Check sheet for the modelled part. Datum: model origin and axes. Units: mm. A direction names the side the tool comes from. Round coordinates to 2 decimals unless told otherwise and drop trailing zeros. Loops run counter-clockwise (first coordinate to the right, second up) from the corner with the lowest first, then second, coordinate; pieces in that order, holes last. Notation, with made-up numbers: (-35, 10) -> (-29, 10) arc R17 ccw to (-29, 26) -> close; hole circle Ø5 at (35, 13). An arc over 180 degrees is marked (long way). Use one line per item in the form item = value. Start each with the question number.
(1) Sectioned sample at A-A (y = -32.5). Record the cut outline in (x, z), and give its area (3 significant figures).
(2) Material ranges on probe 1 along X at (y, z) = (33.5, 11.75); probe 2 along Z at (x, y) = (-32.65, 36); probe 3 along Y at (x, z) = (-33.05, 14.85), recorded low to high. Write a range as [from, to].
(3) Sectioned sample at C-C (y = 39.5). Record the cut outline in (x, z), and give its area (3 significant figures).
(4) Draft check along Y on faces 1 (the flat face through (33.5, -1, 12)), 2 (the flat face through (-31.5, -1, 13)), 3 (the flat face through (0, -65, 12)). Enter one of: released by +Y, released by -Y, zero draft, split by the parting line, or undercut.
(5) Go/stop test with a flat-tipped pin: pin 1 (0.6 mm diameter, centred on y = -64.5, z = 9.5, fed in from +X). Record where the tip stops, or that it passes through.
(6) Sectioned sample at B-B (x = -2). Record the cut outline in (y, z).
(7) Sectioned sample at D-D (x = 27). Record the cut outline in (y, z), and give its area (3 significant figures).
(8) Set-up check for faces 4 (the cylindrical face through (-32.5, -50.6, 13.8)), 5 (the flat face through (0, 63, 13)), 6 (the flat face through (31, 0, 0)): record each of +Z, -Z, +X, -X, +Y, -Y from which the full face is reachable in a straight line by a thin tool's end or side.
from build123d import *

# Parameters (mm, degrees)
SCHIZZO1_W                    = 67
SCHIZZO1_H                    = 130
ESTRUSIONE_ESTRUSIONE1_DEPTH  = 23
SCHIZZO2_W                    = 63
SCHIZZO2_H                    = 126
TAGLIO_ESTRUSIONE1_DEPTH      = 21
TAGLIO_ESTRUSIONE2_DEPTH      = 77.08054942
TAGLIO_ESTRUSIONE2_DEPTH_BACK = 77.08054942
SCHIZZO3_W                    = 59
SCHIZZO3_H                    = 122
TAGLIO_ESTRUSIONE4_REACH      = 98.141
SCHIZZO4_R                    = 1.5
SCHIZZO4_R_2                  = 3.5
SCHIZZO4_R_3                  = 1
SCHIZZO4_W                    = 9
SCHIZZO4_H                    = 15.14
SCHIZZO4_W_2                  = 3.83
SCHIZZO4_H_2                  = 8.75
TAGLIO_ESTRUSIONE5_REACH      = 138.203
SCHIZZO5_W                    = 13
SCHIZZO5_H                    = 3
RACCORDO1_R                   = 1
TAGLIO_ESTRUSIONE6_REACH      = 98.141
SCHIZZO6_R                    = 0.5
SCHIZZO7_R                    = 0.5
TAGLIO_ESTRUSIONE7_DEPTH      = 10
SCHIZZO8_R                    = 0.5
TAGLIO_ESTRUSIONE8_DEPTH      = 10
SCHIZZO9_R                    = 0.54
TAGLIO_ESTRUSIONE9_DEPTH      = 10


with BuildPart() as part:
    # Schizzo1 → Estrusione-Estrusione1 (new body)
    with BuildSketch(Plane.XY):
        Rectangle(SCHIZZO1_W, SCHIZZO1_H)
    extrude(amount=ESTRUSIONE_ESTRUSIONE1_DEPTH)

    # Schizzo2 → Taglio-Estrusione1 (cut)
    with BuildSketch(Plane.XY.offset(23)):
        Rectangle(SCHIZZO2_W, SCHIZZO2_H)
    extrude(amount=-TAGLIO_ESTRUSIONE1_DEPTH, mode=Mode.SUBTRACT)

    # Schizzo3 → Taglio-Estrusione2 (cut, two sides: drawn at the far end of the back side and taken through both)
    with BuildSketch(Plane.XY.offset(2).offset(-TAGLIO_ESTRUSIONE2_DEPTH_BACK)):
        Rectangle(SCHIZZO3_W, SCHIZZO3_H)
    extrude(amount=TAGLIO_ESTRUSIONE2_DEPTH + TAGLIO_ESTRUSIONE2_DEPTH_BACK, mode=Mode.SUBTRACT)

    # Schizzo4 → Taglio-Estrusione4 (cut, up to next)
    with BuildSketch(Plane.ZY.offset(33.5), mode=Mode.PRIVATE) as taglio_estrusione4_sk1:
        with Locations((15, -49.7)):
            Circle(SCHIZZO4_R)
    taglio_estrusione4_tool1 = extrude(taglio_estrusione4_sk1.sketch, amount=-TAGLIO_ESTRUSIONE4_REACH, mode=Mode.PRIVATE) & part.part
    # Schizzo4 → Taglio-Estrusione4 (cut, up to next)
    with BuildSketch(Plane.ZY.offset(33.5), mode=Mode.PRIVATE) as taglio_estrusione4_sk2:
        with Locations((14.85, -19.5)):
            Circle(SCHIZZO4_R_2)
    taglio_estrusione4_tool2 = extrude(taglio_estrusione4_sk2.sketch, amount=-TAGLIO_ESTRUSIONE4_REACH, mode=Mode.PRIVATE) & part.part
    # Schizzo4 → Taglio-Estrusione4 (cut, up to next)
    with BuildSketch(Plane.ZY.offset(33.5), mode=Mode.PRIVATE) as taglio_estrusione4_sk3:
        with Locations((16.2, -44.99254441)):
            Circle(SCHIZZO4_R_3)
    taglio_estrusione4_tool3 = extrude(taglio_estrusione4_sk3.sketch, amount=-TAGLIO_ESTRUSIONE4_REACH, mode=Mode.PRIVATE) & part.part
    # Schizzo4 → Taglio-Estrusione4 (cut, up to next)
    with BuildSketch(Plane.ZY.offset(33.5), mode=Mode.PRIVATE) as taglio_estrusione4_sk4:
        with Locations((16.2, -35.07)):
            Rectangle(SCHIZZO4_W, SCHIZZO4_H)
    taglio_estrusione4_tool4 = extrude(taglio_estrusione4_sk4.sketch, amount=-TAGLIO_ESTRUSIONE4_REACH, mode=Mode.PRIVATE) & part.part
    # Schizzo4 → Taglio-Estrusione4 (cut, up to next)
    with BuildSketch(Plane.ZY.offset(33.5), mode=Mode.PRIVATE) as taglio_estrusione4_sk5:
        with Locations((13.915, -5.715)):
            Rectangle(SCHIZZO4_W_2, SCHIZZO4_H_2)
    taglio_estrusione4_tool5 = extrude(taglio_estrusione4_sk5.sketch, amount=-TAGLIO_ESTRUSIONE4_REACH, mode=Mode.PRIVATE) & part.part
    add(taglio_estrusione4_tool1.solids().sort_by_distance((-33.5, -49.7, 15))[0], mode=Mode.SUBTRACT)
    add(taglio_estrusione4_tool2.solids().sort_by_distance((-33.5, -19.5, 14.85))[0], mode=Mode.SUBTRACT)
    add(taglio_estrusione4_tool3.solids().sort_by_distance((-33.5, -44.992544, 16.2))[0], mode=Mode.SUBTRACT)
    add(taglio_estrusione4_tool4.solids().sort_by_distance((-33.5, -35.07, 16.2))[0], mode=Mode.SUBTRACT)
    add(taglio_estrusione4_tool5.solids().sort_by_distance((-33.5, -5.715, 13.915))[0], mode=Mode.SUBTRACT)

    # Schizzo5 → Taglio-Estrusione5 (cut, up to next)
    with BuildSketch(Plane.XZ.offset(65), mode=Mode.PRIVATE) as taglio_estrusione5_sk1:
        with Locations((-5.741459814, 10)):
            Rectangle(SCHIZZO5_W, SCHIZZO5_H)
    taglio_estrusione5_tool1 = extrude(taglio_estrusione5_sk1.sketch, amount=-TAGLIO_ESTRUSIONE5_REACH, mode=Mode.PRIVATE) & part.part
    add(taglio_estrusione5_tool1.solids().sort_by_distance((-5.74146, -65, 10))[0], mode=Mode.SUBTRACT)

    # Raccordo1
    raccordo1_edges = [part.edges().sort_by_distance(p)[0] for p in [
        (29.5, 0, 0),
        (0, -61, 0),
        (-29.5, 0, 0),
        (0, 61, 0),
        (0, -65, 0),
        (-33.5, 0, 0),
        (0, 65, 0),
        (33.5, 0, 0),
        (33.5, -65, 11.5),
        (-33.5, -65, 11.5),
        (-33.5, 65, 11.5),
        (33.5, 65, 11.5),
    ]]
    fillet(raccordo1_edges, radius=RACCORDO1_R)

    # Schizzo6 → Taglio-Estrusione6 (cut, up to next)
    with BuildSketch(Plane(origin=(33.5, 0, 0), x_dir=(0, 0, -1), z_dir=(1, 0, 0)), mode=Mode.PRIVATE) as taglio_estrusione6_sk1:
        with Locations(Location((-14, -26, 0), (0, 0, 90))):
            Circle(SCHIZZO6_R)
    taglio_estrusione6_tool1 = extrude(taglio_estrusione6_sk1.sketch, amount=-TAGLIO_ESTRUSIONE6_REACH, mode=Mode.PRIVATE) & part.part
    add(taglio_estrusione6_tool1.solids().sort_by_distance((33.5, -26, 14))[0], mode=Mode.SUBTRACT)

    # Schizzo7 → Taglio-Estrusione7 (cut)
    with BuildSketch(Plane(origin=(0, 65, 0), x_dir=(1, 0, 0), z_dir=(0, 1, 0))):
        with Locations(Location((3.81, -14, 0), (0, 0, 270))):
            Circle(SCHIZZO7_R)
    extrude(amount=-TAGLIO_ESTRUSIONE7_DEPTH, mode=Mode.SUBTRACT)

    # Schizzo8 → Taglio-Estrusione8 (cut)
    with BuildSketch(Plane.ZY.offset(33.5)):
        with Locations((14, 36)):
            Circle(SCHIZZO8_R)
    extrude(amount=-TAGLIO_ESTRUSIONE8_DEPTH, mode=Mode.SUBTRACT)

    # Schizzo9 → Taglio-Estrusione9 (cut)
    with BuildSketch(Plane.XZ.offset(65)):
        with Locations(Location((20.5, 14, 0), (0, 0, 270))):
            Circle(SCHIZZO9_R)
    extrude(amount=-TAGLIO_ESTRUSIONE9_DEPTH, mode=Mode.SUBTRACT)


solid = part.part
Checks:
q1.outline = (-33.5, 1) arc R1 ccw to (-32.5, 0) -> (-30.5, 0) arc R1 ccw to (-29.5, 1) -> (-29.5, 2) -> (-31.5, 2) -> (-31.5, 11.7) -> (-33.5, 11.7) -> close; (-33.5, 20.7) -> (-31.5, 20.7) -> (-31.5, 23) -> (-33.5, 23) -> close; (29.5, 1) arc R1 ccw to (30.5, 0) -> (32.5, 0) arc R1 ccw to (33.5, 1) -> (33.5, 23) -> (31.5, 23) -> (31.5, 2) -> (29.5, 2) -> close
q1.area = 81.1 mm2
q2.probe_1 = [-33.5, -31.5], [31.5, 33.5]
q2.probe_2 = [0.01, 13.5], [14.5, 23]
q2.probe_3 = [-64.84, -51.19], [-48.21, -42.64], [-27.5, -23], [-16, -10.09], [-1.34, 64.84]
q3.outline = (-33.5, 1) arc R1 ccw to (-32.5, 0) -> (-30.5, 0) arc R1 ccw to (-29.5, 1) -> (-29.5, 2) -> (-31.5, 2) -> (-31.5, 23) -> (-33.5, 23) -> close; (29.5, 1) arc R1 ccw to (30.5, 0) -> (32.5, 0) arc R1 ccw to (33.5, 1) -> (33.5, 23) -> (31.5, 23) -> (31.5, 2) -> (29.5, 2) -> close
q3.area = 99.1 mm2
q4.face_1 = zero draft
q4.face_2 = undercut
q4.face_3 = released by -Y
q5.pin_1 = 33.48
q6.outline = (-65, 1) arc R1 ccw to (-64, 0) -> (-62, 0) arc R1 ccw to (-61, 1) -> (-61, 2) -> (-63, 2) -> (-63, 8.5) -> (-65, 8.5) -> close; (-65, 11.5) -> (-63, 11.5) -> (-63, 23) -> (-65, 23) -> close; (61, 1) arc R1 ccw to (62, 0) -> (64, 0) arc R1 ccw to (65, 1) -> (65, 23) -> (63, 23) -> (63, 2) -> (61, 2) -> close
q7.outline = (-65, 1) arc R1 ccw to (-64, 0) -> (-62, 0) arc R1 ccw to (-61, 1) -> (-61, 2) -> (-63, 2) -> (-63, 23) -> (-65, 23) -> close; (61, 1) arc R1 ccw to (62, 0) -> (64, 0) arc R1 ccw to (65, 1) -> (65, 23) -> (63, 23) -> (63, 2) -> (61, 2) -> close
q7.area = 99.1 mm2
q8.face_4 = -X
q8.face_5 = +Z
q8.face_6 = -Z, +X, -X, +Y, -Y
